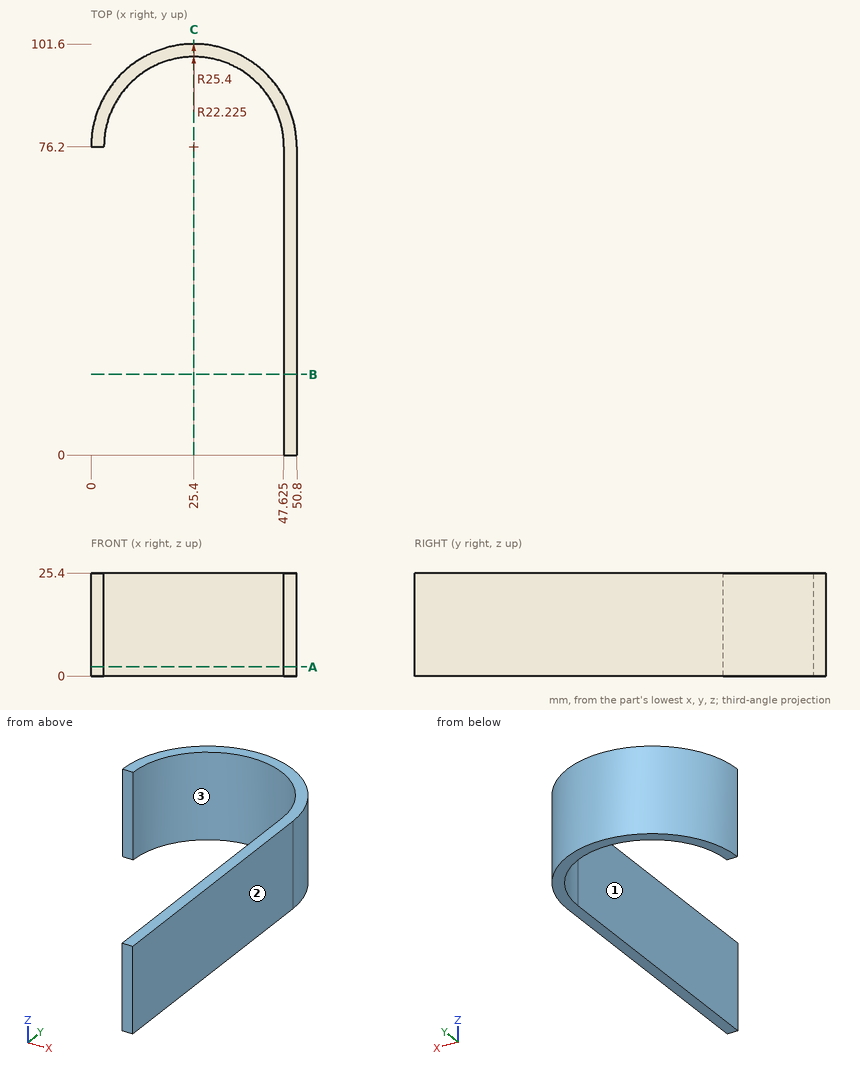
Drawing for the job (mm, zero at the part's lowest x, y, z). Coordinates: 2 decimals unless noted, no trailing zeros. Write each loop counter-clockwise with the first axis right and the second up, starting at its lowest first coordinate (ties: lowest second). Pieces come first, ordered by that corner, then holes. Notation, with made-up numbers: (9.25, -40) - (49.25, -40) arc R11 ccw to (49.25, -28) - close; hole circle Ø4 at (-5, 79.25). An arc over 180 degrees is marked (long way). Write each question's results on one line, items separated by ' | '. Start each with the question number.
1) Flat gauge pins, fed straight in: P1, Ø3, axis at x = 38, z = 9.5, coming from the +Y side; P2, Ø1, axis at x = 31, z = 13.5, coming from the -Y side; P3, Ø1, axis at x = 1.5, z = 10, coming from the -Y side; P4, Ø1.5, axis at y = 77, z = 15, coming from the -X side. Where does each tip first touch, or does it go through?
2) Cut at B-B (y = 20). Write the cut outline in (x, z) (3 decimals).
3) Cut at C-C (x = 25.4). Write the cut outline in (y, z) (3 decimals), then the cut area to 3 significant figures.
4) Mould opens along X. For the marked faces 1, 2 and 3 say: pulls with the +X half, pulls with the -X half, needs draft (parallel to the pull), parting line crosses it, or undercut.
5) Cut at A-A (z = 2.25). Write the cut outline in (x, y) (3 decimals).
6) Probe line 1 along X through (y, z) = (27, 9.25) (3 decimals); line 2 along Y through (x, z) = (37, 8.25); line 3 along Y through (x, z) = (8, 13.75). List the from-to ranges inside material, lowest first. Write a range as from..to.
Returned:
1) P1: y = 99.05 | P2: y = 97.57 | P3: y = 76.2 | P4: x = 0
2) outline: (47.625, 0) - (50.8, 0) - (50.8, 25.4) - (47.625, 25.4) - close
3) outline: (98.425, 0) - (101.6, 0) - (101.6, 25.4) - (98.425, 25.4) - close | area: 80.6 mm^2
4) face 1: pulls with the -X half | face 2: pulls with the +X half | face 3: undercut
5) outline: (0, 76.2) - (3.175, 76.2) arc R22.225 cw to (47.625, 76.2) - (47.625, 0) - (50.8, 0) - (50.8, 76.2) arc R25.4 ccw to start
6) line 1: 47.625..50.8 | line 2: 95.16..98.8 | line 3: 90.03..94.7
